Geometry check sheet. Reference: the model listing, model coordinates, mm. A direction names the side the tool comes from. Coordinates: 2 decimals unless noted, no trailing zeros. Loops run counter-clockwise (first coordinate to the right, second up) from the corner with the lowest first, then second, coordinate; pieces in that order, holes last.
from build123d import *

# Parameters (mm, degrees)
PAD_DEPTH         = 20
SKETCH001_R       = 2.5
POCKET_DEPTH      = 80.001
POCKET_DEPTH_BACK = -0.001


with BuildPart() as part:
    # Sketch → Pad (new body, symmetric)
    with BuildSketch(Plane.XY):
        Polygon((-40, 60), (-20, 60), (-20, 15), (20, 15), (20, 60), (40, 60), (40, -60), (20, -60), (20, -15), (-20, -15), (-20, -60), (-40, -60), align=None)
    extrude(amount=PAD_DEPTH, both=True)

    # Sketch001 → Pocket (cut, two sides)
    with BuildSketch(Plane.YZ.offset(40)) as pocket_sk:
        with Locations((-40, 0)):
            Circle(SKETCH001_R)
        with Locations((40, 0)):
            Circle(SKETCH001_R)
    extrude(amount=-POCKET_DEPTH, mode=Mode.SUBTRACT)
    extrude(pocket_sk.sketch, amount=-POCKET_DEPTH_BACK, mode=Mode.SUBTRACT)


solid = part.part
(1) Sectioned sample at C-C on y = -40. Record the cut outline in (x, z), and give its area (3 significant figures).
Findings:
outline: (-40, -20) - (-20, -20) - (-20, -2.5) - (-40, -2.5) - close; (-40, 2.5) - (-20, 2.5) - (-20, 20) - (-40, 20) - close; (20, -20) - (40, -20) - (40, -2.5) - (20, -2.5) - close; (20, 2.5) - (40, 2.5) - (40, 20) - (20, 20) - close
area: 1,400 mm2
(2) Sectioned sample at A-A on z = 0. Record the cut outline in (x, y), and give its area (3 significant figures).
Findings:
outline: (-40, -60) - (-20, -60) - (-20, -42.5) - (-40, -42.5) - close; (-40, -37.5) - (-20, -37.5) - (-20, -15) - (20, -15) - (20, -37.5) - (40, -37.5) - (40, 37.5) - (20, 37.5) - (20, 15) - (-20, 15) - (-20, 37.5) - (-40, 37.5) - close; (-40, 42.5) - (-20, 42.5) - (-20, 60) - (-40, 60) - close; (20, -60) - (40, -60) - (40, -42.5) - (20, -42.5) - close; (20, 42.5) - (40, 42.5) - (40, 60) - (20, 60) - close
area: 5,600 mm2
(3) Scan lines: L1, parallel to X at y = 31.5, z = 17; L2, parallel to Z at x = 26.5, y = 40; L3, parallel to Y at x = -12, z = -1. Record each from-to range of solid material in increasing order.
Findings:
L1: x = -40 to -20, 20 to 40
L2: z = -20 to -2.5, 2.5 to 20
L3: y = -15 to 15
(4) Sectioned sample at D-D on x = 2. Record the cut outline in (y, z).
Findings:
outline: (-15, -20) - (15, -20) - (15, 20) - (-15, 20) - close
(5) Sectioned sample at B-B on y = 44. Record the cut outline in (x, z), and give its area (3 significant figures).
Findings:
outline: (-40, -20) - (-20, -20) - (-20, 20) - (-40, 20) - close; (20, -20) - (40, -20) - (40, 20) - (20, 20) - close
area: 1,600 mm2
(6) Gauge pin test, flat ends, axial feed: pin 1 Ø4.5 at (y, z) = (-40, 0) entering from -X; pin 2 Ø4 at (x, z) = (3.5, -14.5) entering from -Y; pin 3 Ø3 at (x, z) = (-1.5, -5.5) entering from +Y. Record the tip position at first contact, or that the pin passes through.
Findings:
pin 1: passes through
pin 2: stops at y = -15
pin 3: stops at y = 15
(7) Draft check along Y on faces 4 (the flat face through (-20, 38, 5)), 5 (the cylindrical face through (-29.86, 42.31, -0.96)), 6 (the flat face through (-30, 60, 0)). Enter one of: +Y half, -Y half, draft (parallel to the pull), parting line (faces both ways), or undercut.
Findings:
face 4: draft
face 5: undercut
face 6: +Y half
(8) Access from +Z, -Z, +X, -X, +Y, -Y to the whole of each face (thin tool, end or side, straight path). Record for faces 1 (the flat face through (40, 1, 0)), 2 (the flat face through (20, -38, 5)), 3 (the flat face through (0, 15, 0)).
Findings:
face 1: +Z, -Z, +X, +Y, -Y
face 2: +Z, -Z, -Y
face 3: +Z, -Z, +Y
